Read the model definition and answer for the solid it produces. Units are mm, in the model's axes. Face numbers are marked on the shaded views. Round coordinates to 2 decimals unless told otherwise and drop trailing zeros. Loops run counter-clockwise (first coordinate to the right, second up) from the corner with the lowest first, then second, coordinate; pieces in that order, holes last. Notation, with made-up numbers: M 88.25,-2 L 101.25,-2 A13 cw 101.25,7 Z; hole C 53,63 d10. An arc over 180 degrees is marked long. Write each question's results on one line, items separated by ' | '.
from build123d import *

# Parameters (mm, degrees)
CYLINDER_R     = 2
CYLINDER_DEPTH = 10
BOX_W          = 5
BOX_H          = 17
BOX_DEPTH      = 5
BOX001_W       = 13
BOX001_H       = 20.5
BOX001_DEPTH   = 10
FILLET_R       = 2


with BuildPart() as cylinder:
    # Cylinder → Cylinder (new body)
    with BuildSketch(Plane(origin=(9, 10.25, 0), x_dir=(1, 0, 0), z_dir=(0, 0, 1))):
        Circle(CYLINDER_R)
    extrude(amount=CYLINDER_DEPTH)


with BuildPart() as cube:
    # Box → Box (new body)
    with BuildSketch(Plane(origin=(0, 1.5, 5), x_dir=(1, 0, 0), z_dir=(0, 0, 1))):
        with Locations((2.5, 8.5)):
            Rectangle(BOX_W, BOX_H)
    extrude(amount=BOX_DEPTH)


with BuildPart() as fillet_body:
    # Box001 → Box001 (new body)
    with BuildSketch(Plane.XY):
        with Locations((6.5, 10.25)):
            Rectangle(BOX001_W, BOX001_H)
    extrude(amount=BOX001_DEPTH)

    # Cut: cut Cube
    add(cube.part, mode=Mode.SUBTRACT)

    # Cut001: cut Cylinder
    add(cylinder.part, mode=Mode.SUBTRACT)

    # Fillet
    fillet_edges = [fillet_body.edges().sort_by_distance(p)[0] for p in [
        (13, 20.5, 5),
        (13, 0, 5),
    ]]
    fillet(fillet_edges, radius=FILLET_R)


solid = fillet_body.part
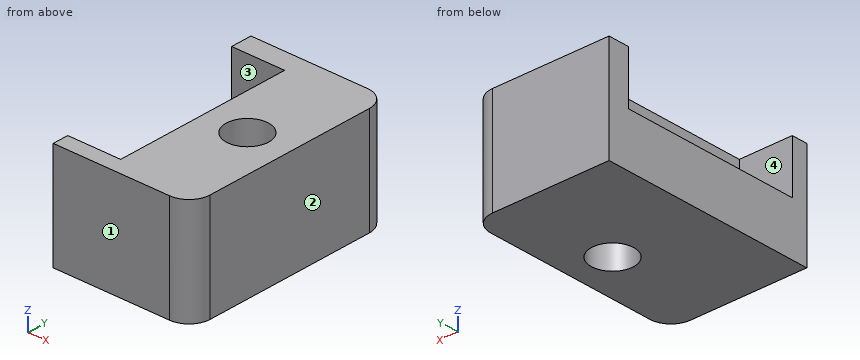
Item 1: The mould has two halves that part along Y. Classify the marked faces 1, 2, 3 and 4: pulls with the +Y half, pulls with the -Y half, needs draft (parallel to the pull), parting line crosses it, or undercut.
Outcome:
face 1: pulls with the -Y half | face 2: needs draft | face 3: undercut | face 4: undercut
Item 2: The part is cut by section A-A (y = 10.25). Determine the outline of the cut face in (x, z).
Outcome:
outline: M 0,0 L 7,0 L 7,10 L 5,10 L 5,5 L 0,5 Z; M 11,0 L 13,0 L 13,10 L 11,10 Z
Item 3: The part is cut by section B-B (x = 9). Determine the outline of the cut face in (y, z), plus the area to 3 significant figures.
Outcome:
outline: M 0,0 L 8.25,0 L 8.25,10 L 0,10 Z; M 12.25,0 L 20.5,0 L 20.5,10 L 12.25,10 Z | area: 165 mm2
Item 4: A flat-ended cylindrical pin translates along its axis: pin 1 (4 mm diameter, centred on y = 13, z = 8, fed in from -X). Find the tip coordinate at first contact, or state that the pin passes through.
Outcome:
pin 1: stops at x = 5
Item 5: The part is cut by section D-D (y = 16). Determine the outline of the cut face in (x, z), plus the area to 3 significant figures.
Outcome:
outline: M 0,0 L 13,0 L 13,10 L 5,10 L 5,5 L 0,5 Z | area: 105 mm2
Item 6: The part is cut by section C-C (z = 2.5). Determine the outline of the cut face in (x, y).
Outcome:
outline: M 0,0 L 11,0 A2 ccw 13,2 L 13,18.5 A2 ccw 11,20.5 L 0,20.5 Z; hole C 9,10.25 d4
Item 7: Straight lines are drawn through the part: line 1 (Y direction, x = 9, z = 2.5); line 2 (Z direction, x = 2, y = 8); line 3 (Y direction, x = 7.5, z = 1). For each, find the intervals that lie inside material, in ascending order.
Outcome:
line 1: y = 0 to 8.25, 12.25 to 20.5 | line 2: z = 0 to 5 | line 3: y = 0 to 8.93, 11.57 to 20.5
